from build123d import *

# Parameters (mm, degrees)
SKETCH1_W                = 20
SKETCH1_H                = 350
BOSS_EXTRUDE1_DEPTH      = 10
BOSS_EXTRUDE1_2_DEPTH    = 10
BOSS_EXTRUDE2_DEPTH      = 0.001
BOSS_EXTRUDE2_DEPTH_BACK = 10
SKETCH2_W                = 107.015982705
SKETCH2_H                = 50
SKETCH3_W                = 120
SKETCH3_H                = 200
BOSS_EXTRUDE3_DEPTH      = 3
SKETCH4_W                = 120
SKETCH4_H                = 4
BOSS_EXTRUDE4_DEPTH      = 150
SKETCH5_R                = 40
CUT_EXTRUDE1_DEPTH       = 90
BOSS_EXTRUDE5_DEPTH      = 90
BOSS_EXTRUDE5_DEPTH_BACK = 70
SKETCH6_R                = 40
SKETCH7_R                = 38
CUT_EXTRUDE2_DEPTH       = 176
SKETCH8_W                = 20
SKETCH8_H                = 10
SKETCH8_W_2              = 23
BOSS_EXTRUDE6_DEPTH      = 70
SKETCH9_W                = 470.324280976
SKETCH9_H                = 9.538817488
BOSS_EXTRUDE7_DEPTH      = 400
SKETCH10_W               = 511.33
SKETCH10_H               = 10
BOSS_EXTRUDE8_DEPTH      = 180
SKETCH11_W               = 160
SKETCH11_H               = 60
BOSS_EXTRUDE9_DEPTH      = 120


with BuildPart() as part:
    # Sketch1 → Boss-Extrude1 (new body)
    with BuildSketch(Plane(origin=(0, 0, 0), x_dir=(1, 0, 0), z_dir=(0, 1, 0))):
        with Locations((-51.819592314, 74.671278777)):
            Rectangle(SKETCH1_W, SKETCH1_H)
    extrude(amount=BOSS_EXTRUDE1_DEPTH)



with BuildPart() as body_2:
    # Sketch1 → Boss-Extrude1 2 (new body)
    with BuildSketch(Plane(origin=(0, 0, 0), x_dir=(1, 0, 0), z_dir=(0, 1, 0))):
        with Locations((36.510407686, 74.671278777)):
            Rectangle(SKETCH1_W, SKETCH1_H)
    extrude(amount=BOSS_EXTRUDE1_2_DEPTH)


with BuildPart() as part_1:
    add(part.part)

    add(body_2.part)  # Boss-Extrude2 merges body 2
    # Sketch2 → Boss-Extrude2 (add, two sides: drawn at the far end of the back side and taken through both)
    with BuildSketch(Plane(origin=(0, 0, 0), x_dir=(-1, 0, 0), z_dir=(0, -1, 0)).offset(-BOSS_EXTRUDE2_DEPTH_BACK)):
        with Locations((6.997583667, 274.671278777)):
            Rectangle(SKETCH2_W, SKETCH2_H)
    extrude(amount=BOSS_EXTRUDE2_DEPTH + BOSS_EXTRUDE2_DEPTH_BACK)

    # Sketch3 → Boss-Extrude3 (add)
    with BuildSketch(Plane(origin=(46.510407686, 0, 0), x_dir=(0, 0, -1), z_dir=(1, 0, 0))):
        with Locations((-40.328721223, 100)):
            Rectangle(SKETCH3_W, SKETCH3_H)
    extrude(amount=BOSS_EXTRUDE3_DEPTH)

    # Sketch4 → Boss-Extrude4 (add)
    with BuildSketch(Plane.ZY.offset(-46.510407686)):
        with Locations((40.328721223, 158)):
            Rectangle(SKETCH4_W, SKETCH4_H)
        with Locations((40.328721223, 118)):
            Rectangle(SKETCH4_W, SKETCH4_H)
    extrude(amount=BOSS_EXTRUDE4_DEPTH)

    # Sketch5 → Cut-Extrude1 (cut)
    with BuildSketch(Plane(origin=(0, 160, 0), x_dir=(1, 0, 0), z_dir=(0, 1, 0))):
        with Locations(Location((-8.489592314, -37.781336818, 0), (0, 0, 270))):
            Circle(SKETCH5_R)
    extrude(amount=-CUT_EXTRUDE1_DEPTH, mode=Mode.SUBTRACT)

    # Sketch6 → Boss-Extrude5 (add, two sides: drawn at the far end of the back side and taken through both)
    with BuildSketch(Plane(origin=(0, 160, 0), x_dir=(1, 0, 0), z_dir=(0, 1, 0)).offset(-BOSS_EXTRUDE5_DEPTH_BACK)):
        with Locations(Location((-8.489592314, -37.781336818, 0), (0, 0, 270))):
            Circle(SKETCH6_R)
    extrude(amount=BOSS_EXTRUDE5_DEPTH + BOSS_EXTRUDE5_DEPTH_BACK)

    # Sketch7 → Cut-Extrude2 (cut)
    with BuildSketch(Plane(origin=(0, 250, 0), x_dir=(1, 0, 0), z_dir=(0, 1, 0))):
        with Locations(Location((-8.489592314, -37.781336818, 0), (0, 0, 270))):
            Circle(SKETCH7_R)
    extrude(amount=-CUT_EXTRUDE2_DEPTH, mode=Mode.SUBTRACT)

    # Sketch8 → Boss-Extrude6 (add)
    with BuildSketch(Plane.XY.offset(100.328721223)):
        with Locations((-51.819592314, 5)):
            Rectangle(SKETCH8_W, SKETCH8_H)
        with Locations((38.010407686, 5)):
            Rectangle(SKETCH8_W_2, SKETCH8_H)
    extrude(amount=BOSS_EXTRUDE6_DEPTH)

    # Sketch9 → Boss-Extrude7 (add)
    with BuildSketch(Plane(origin=(49.510407686, 0, 0), x_dir=(0, 0, -1), z_dir=(1, 0, 0))):
        with Locations((64.833419265, 5.230591256)):
            Rectangle(SKETCH9_W, SKETCH9_H)
    extrude(amount=BOSS_EXTRUDE7_DEPTH)

    # Sketch10 → Boss-Extrude8 (add)
    with BuildSketch(Plane.XY.offset(170.328721223)):
        with Locations((193.845407686, 5)):
            Rectangle(SKETCH10_W, SKETCH10_H)
    extrude(amount=BOSS_EXTRUDE8_DEPTH)

    # Sketch11 → Boss-Extrude9 (add)
    with BuildSketch(Plane(origin=(0, 10, 0), x_dir=(1, 0, 0), z_dir=(0, 1, 0))):
        with Locations((18.180407686, -252.921925031)):
            Rectangle(SKETCH11_W, SKETCH11_H)
    extrude(amount=BOSS_EXTRUDE9_DEPTH)


solid = part_1.part
Can you work these out from the model? Positions are in its coordinate system, mm. A direction names the side the tool comes from. Round coordinates to 2 decimals unless told otherwise and drop trailing zeros. Write each loop counter-clockwise with the first axis right and the second up, starting at its lowest first coordinate (ties: lowest second). Pieces come first, ordered by that corner, then holes. Notation, with made-up numbers: (73.5, 19) -> (104.5, 19) arc R6 ccw to (104.5, 27) -> close; hole circle Ø10 at (88.25, 37.5). An arc over 180 degrees is marked (long way). Use one line per item in the form item = value. Start each with the question number.
Q1. Imagine slicing it at D-D (z = 117). Please give me the cut outline in (x, y).
Q2. Imagine slicing it at C-C (x = 63.5). Please give me the cut outline in (y, z), then the cut area to 3 significant figures.
Q3. Imagine slicing it at B-B (y = 82). Please give me the cut outline in (x, z), then the cut area to 3 significant figures.
Q4. If I drill on probe 1 along Y at (x, z) = (-55, 100); probe 2 along Y at (x, z) = (270.5, 112.5); probe 3 along Z at (x, y) = (-39, 110.5), over which ranges is the centre line in solid material (lowest first)? Write a range as [from, to].
Q5. Which directions (+Z, -Z, +X, -X, +Y, -Y) give clear straight access to the entire face, cutting with the end or side of a thin tool? Please do faces 1 (the face through (17, 69, 222.922)), 2 (the face through (-23.1, 90, 73.2)), 3 (the face through (-61, 156, 39)).
Q6. Imagine slicing it at A-A (z = -69.5). Please give me the cut outline in (x, y), then the cut area to 3 significant figures.
Q7. We'd pull the mould along Z, two halves only. Please class faces 4 (the face through (46.51, 64, 41)), 5 (the face through (-61, 116, 39)), 6 (the face through (-27, 159, -19.671)): +Z half, -Z half, draft (parallel to the pull), parting line (faces both ways), or undercut.
Q8. I'm going to push flat-ended pins straight in: P1, Ø2, axis at y = 78.5, z = 60.5, coming from the +X side; P2, Ø8, axis at x = 168, z = 238.5, coming from the -Y side; P3, Ø12, axis at y = 189, z = 35, coming from the -X side; P4, Ø1.5, axis at x = -1.5, y = 79.5, coming from the +Z side. Where does each tip first touch, or does it pass through?
Worked out:
q1.outline = (-61.82, 0) -> (-41.82, 0) -> (-41.82, 10) -> (-61.82, 10) -> close; (26.51, 0) -> (49.51, 0) -> (49.51, 0.46) -> (449.51, 0.46) -> (449.51, 10) -> (26.51, 10) -> close
q2.outline = (0, 170.33) -> (0.46, 170.33) -> (0.46, -300) -> (10, -300) -> (10, 222.92) -> (130, 222.92) -> (130, 282.92) -> (10, 282.92) -> (10, 350.33) -> (0, 350.33) -> close
q2.area = 13,500 mm^2
q3.outline = (-61.82, 222.92) -> (98.18, 222.92) -> (98.18, 282.92) -> (-61.82, 282.92) -> close; (46.51, -19.67) -> (49.51, -19.67) -> (49.51, 100.33) -> (46.51, 100.33) -> close
q3.area = 9,960 mm^2
q4.probe_1 = [0, 10], [116, 120], [156, 160]
q4.probe_2 = [0.46, 10]
q4.probe_3 = [11.91, 15.13], [60.43, 63.65], [222.92, 282.92]
q5.face_1 = +X, -X, +Y
q5.face_2 = -Z, -X
q5.face_3 = none
q6.outline = (-61.82, 0) -> (-41.82, 0) -> (-41.82, 10) -> (-61.82, 10) -> close; (26.51, 0) -> (46.51, 0) -> (46.51, 10) -> (26.51, 10) -> close; (49.51, 0.46) -> (449.51, 0.46) -> (449.51, 10) -> (49.51, 10) -> close
q6.area = 4,220 mm^2
q7.face_4 = draft
q7.face_5 = undercut
q7.face_6 = -Z half
q8.P1 = 49.51
q8.P2 = 0
q8.P3 = -48.49
q8.P4 = 282.92
